Autodesk Inventor part; units mm, degrees
ref_plane "YZ Plane" through (0, 0, 0) normal (1, 0, 0) x (0, 1, 0)
ref_plane "XZ Plane" through (0, 0, 0) normal (0, 1, 0) x (-1, 0, 0)
ref_plane "XY Plane" through (0, 0, 0) normal (0, 0, 1) x (1, 0, 0)
sketch "Sketch1" plane through (0, 0, 0) normal (0, 0, 1) x (1, 0, 0)
  line L0 (-20.5422, 8) -> (20.5422, 8)
  line L1 (20.5422, 8) -> (20.5422, -12)
  line L2 (20.5422, -12) -> (-20.5422, -12)
  line L3 (-20.5422, -12) -> (-20.5422, 8)
  arc A0 (-13, -4.0277) -> (-15, -4.0277) centre (-14, 0) ccw
  arc A1 (15, -4.0277) -> (13, -4.0277) centre (14, 0) ccw
  line L4 (0, 8) -> (0, -12) construction
  line L5 (-13, -4.0277) -> (-13, -12)
  line L6 (-13, -12) -> (-15, -12)
  line L7 (-15, -12) -> (-15, -4.0277)
  line L8 (15, -4.0277) -> (15, -12)
  line L9 (15, -12) -> (13, -12)
  line L10 (13, -12) -> (13, -4.0277)
  line L11 (-20.5422, -4) -> (-18, -4)
  line L12 (-18, -4) -> (-18, -12)
  line L13 (-18, -12) -> (-20.5422, -12)
  line L14 (-20.5422, -12) -> (-20.5422, -4)
  line L15 (18, -4) -> (20.5422, -4)
  line L16 (20.5422, -4) -> (20.5422, -12)
  line L17 (20.5422, -12) -> (18, -12)
  line L18 (18, -12) -> (18, -4)
  line L19 (-8.5, -4) -> (8.5, -4)
  line L20 (8.5, -4) -> (8.5, -12)
  line L21 (8.5, -12) -> (-8.5, -12)
  line L22 (-8.5, -12) -> (-8.5, -4)
  line L23 (-8.5, 8) -> (8.5, 8)
  line L24 (8.5, 8) -> (8.5, 4)
  line L25 (8.5, 4) -> (-8.5, 4)
  line L26 (-8.5, 4) -> (-8.5, 8)
  point P0 (0, 0)
  point P1 (0, -2)
  point P2 (-14, -4.3116)
  point P3 (14, -4.0277)
  point P4 (0, -4)
  point P5 (-13, -12)
  point P6 (-8.5, -12)
  point P7 (8.5, -12)
  point P8 (20.5422, -4)
  point P9 (8.5, 8)
  point P10 (-8.5, 8)
  point P11 (-15, -12)
  dimension "d0" = 8.3
  dimension "d1" = 28
  dimension "d2" = 2
  dimension "d4" = 2
  dimension "d6" = 41.0844
  dimension "d7" = 8
  dimension "d8" = 12
  dimension "d9" = 20
  dimension "d10" = 3
  dimension "d11" = 3
  dimension "d13" = 8
  dimension "d15" = 5.5
  dimension "d16" = 5.5
  dimension "d17" = 4
  dimension "d18" = 4
extrude "Extrusion1" add sketch "Sketch1" along normal blind 10 contours L0 L26 L25 L24 L1 L15 L18 L2 L8 A1 L10 L20 L19 L22 L5 A0 L7 L12 L11 L3
sketch "Sketch2" plane through (-18, -12, 0) normal (-1, 0, 0) x (0, 0, 1)
  circle A0 centre (5, 4) radius 1.75
  line L0 (0, 0) -> (10, 0)
  line L1 (10, 8) -> (10, 0)
  circle A1 centre (5, 4) radius 3 construction
  point P0 (0, 12)
  point P1 (5, 0)
  point P2 (10, 4)
  dimension "d22" = 3.5
  dimension "d23" = 6
hole "Hole1" at (-18, -8, 5) direction (1, 0, 0) diameter 4 end through all
fillet "Fillet2" radius 0.5 8 edges at (-18, -4, 5) (-8.5, -4, 5) (8.5, -4, 5) (18, -4, 5) (-18, -12, 5) (-8.5, -12, 5) (8.5, -12, 5) (18, -12, 5)
sketch "Sketch4" plane through (0, 0, 10) normal (0, 0, 1) x (1, 0, 0)
  line L0 (-30.5422, 8) -> (-20.5422, 8)
  line L1 (-20.5422, 8) -> (-20.5422, -4)
  line L2 (-20.5422, -4) -> (-30.5422, -4)
  line L3 (-30.5422, -4) -> (-30.5422, 8)
  line L4 (20.5422, 8) -> (30.5422, 8)
  line L5 (30.5422, 8) -> (30.5422, -4)
  line L6 (30.5422, -4) -> (20.5422, -4)
  line L7 (20.5422, -4) -> (20.5422, 8)
  line L8 (20.5422, -4) -> (20.5422, 8)
  line L9 (18.5, -4) -> (20.5422, -4)
  line L10 (20.5422, 8) -> (8.5, 8)
  line L11 (-8.5, 8) -> (-20.5422, 8)
  line L12 (-20.5422, -4) -> (-18.5, -4)
  line L13 (-20.5422, 8) -> (-20.5422, -4)
  circle A0 centre (-25.5422, 2) radius 2.5
  circle A1 centre (25.5422, 2) radius 2.5
  point P0 (0, 0)
  point P1 (25.5422, 8)
  point P2 (30.5422, 2)
  point P3 (-30.5422, 2)
  point P4 (-25.5422, 8)
  dimension "d32" = 10
  dimension "d33" = 5
  dimension "d34" = 0
  dimension "d35" = 0
  dimension "d36" = 0
  dimension "d37" = 0
extrude "Extrusion2" add sketch "Sketch4" against normal up to surface (10 mm away)
fillet "Fillet3" radius 4 8 edges at (8.5, 8, 5) (30.5422, 8, 5) (30.5422, -4, 5) (8.5, 4, 5) (-8.5, 4, 5) (-8.5, 8, 5) (-30.5422, 8, 5) (-30.5422, -4, 5)
equation "\"d4\" = d2"
equation "\"d11\" = d10"
equation "\"d13\" = d7"
properties part number "0008-30-006"
For this review, take the finished solid that the model builds, in its own axes (mm). A direction names the side the tool comes from. Coordinates: 2 decimals unless noted, no trailing zeros. Write each loop counter-clockwise with the first axis right and the second up, starting at its lowest first coordinate (ties: lowest second). Pieces come first, ordered by that corner, then holes.
(1) Add section D-D on y = -2.5. Give the boundary of the cut face in (x, z), then the cut area to 3 significant figures.
(2) For pin 1 Ø6 at (y, z) = (-6, 8) entering from -X; pin 2 Ø3.5 at (y, z) = (-7, 2.5) entering from +X; pin 3 Ø3.5 at (y, z) = (-7, 4) entering from -X; pin 4 Ø4.5 at (x, y) = (-25.54, 2) entering from +Z, all flat-tipped, find the tip position at first contact; note any pin that passes through.
(3) Wall thickness on probe 1 along X at (y, z) = (-4.5, 7); probe 2 along Y at (x, z) = (11.1, 5); probe 3 along Z at (x, y) = (15.8, -8): over which ranges is each line inside the solid? List them lowest first.
(4) Add section B-B on x = -10.5. Give the boundary of the cut face in (y, z), then the cut area to 3 significant figures.
(5) Tool access review of faces 5 (the face through (-11, -12, 5)), 6 (the face through (-18, -8, 2.7)), 7 (the face through (19, 8, 5)), 8 (the face through (22, -4, 5)), 9 (the face through (-8.5, -8, 2.7)): name each direction out of +Z, -Z, +X, -X, +Y, -Y from which nothing blocks a thin tool from reaching the whole face with its end or side.
(6) The part is to be moulded in two halves that separate along Z. For faces 1 (the face through (-14.168, 4.147, 4.93)), 2 (the face through (0, 3, 0)), 3 (the face through (-16.479, -9.352, 3.526)), 4 (the face through (0, 3, 10)), say which applies: +Z half, -Z half, draft (parallel to the pull), parting line (faces both ways), or undercut.
(7) Add section A-A on y = -8. Count the separate pieces of the cut face and the enclosed holes in it, then the cut area to 3 significant figures.
(8) Add section C-C on y = 2. Give the boundary of the cut face in (x, z).
Answer sheet:
1. outline: (-29.66, 0) - (-17.31, 0) - (-17.31, 10) - (-29.66, 10) - close; (-10.69, 0) - (10.69, 0) - (10.69, 10) - (-10.69, 10) - close; (17.31, 0) - (29.66, 0) - (29.66, 10) - (17.31, 10) - close
1. area: 461 mm2
2. pin 1: stops at x = -29.19
2. pin 2: stops at x = 18
2. pin 3: stops at x = -18
2. pin 4: passes through
3. probe 1: x = -18 to -15, -13 to -8.5, 8.5 to 13, 15 to 18
3. probe 2: y = -12 to -10, -6 to -2.97, 2.97 to 7.99
3. probe 3: z = 0 to 3, 7 to 10
4. outline: (-12, 0) - (-2.23, 0) - (-2.23, 10) - (-12, 10) - close; (2.23, 0) - (7.46, 0) - (7.46, 10) - (2.23, 10) - close; hole circle Ø4 at (-8, 5)
4. area: 137 mm2
5. face 5: +Z, -Z, +X, -X, -Y
5. face 6: +Z, -Z, -X, -Y
5. face 7: +Z, -Z, +X, -X, +Y
5. face 8: +Z, -Z, +X, -Y
5. face 9: +Z, -Z, -Y
6. face 1: draft
6. face 2: -Z half
6. face 3: undercut
6. face 4: +Z half
7. separate pieces: 8
7. enclosed holes: 0
7. area: 90.0 mm2
8. outline: (-30.54, 0) - (-28.04, 0) - (-28.04, 10) - (-30.54, 10) - close; (-23.04, 0) - (-17.64, 0) - (-17.64, 10) - (-23.04, 10) - close; (-10.36, 0) - (10.36, 0) - (10.36, 10) - (-10.36, 10) - close; (17.64, 0) - (23.04, 0) - (23.04, 10) - (17.64, 10) - close; (28.04, 0) - (30.54, 0) - (30.54, 10) - (28.04, 10) - close
